from build123d import *

# Parameters (mm, degrees)
SKETCH1_R           = 1.135
SKETCH1_R_2         = 1.054
BOSS_EXTRUDE1_DEPTH = 3
SKETCH2_R           = 0.65
CUT_EXTRUDE1_DEPTH  = 23.736281859
SKETCH4_R           = 0.25
CUT_EXTRUDE3_DEPTH  = 0.25


with BuildPart() as part:
    # Sketch1 → Boss-Extrude1 (new body)
    with BuildSketch(Plane(origin=(0, 0, 0), x_dir=(1, 0, 0), z_dir=(0, 1, 0))):
        with BuildLine():
            Line((0, 0), (9.035898385, 0))
            ThreePointArc((9.035898385, 0), (10.767949192, 1), (10.767949192, 3))
            Line((10.767949192, 3), (1.732050808, 18.650635095))
            ThreePointArc((1.732050808, 18.650635095), (0, 19.650635095), (-1.732050808, 18.650635095))
            Line((-1.732050808, 18.650635095), (-10.767949192, 3))
            ThreePointArc((-10.767949192, 3), (-10.767949192, 1), (-9.035898385, 0))
            Line((-9.035898385, 0), (0, 0))
        make_face()
        with Locations(Location((0, 17.650635095, 0), (0, 0, 270))):
            Circle(SKETCH1_R, mode=Mode.SUBTRACT)
        with Locations(Location((-9.035898385, 2, 0), (0, 0, 270))):
            Circle(SKETCH1_R, mode=Mode.SUBTRACT)
        with Locations(Location((9.035898385, 2, 0), (0, 0, 270))):
            Circle(SKETCH1_R_2, mode=Mode.SUBTRACT)
    extrude(amount=BOSS_EXTRUDE1_DEPTH)

    # Sketch2 → Cut-Extrude1 (cut, through all)
    with BuildSketch(Plane(origin=(0, 3, 0), x_dir=(1, 0, 0), z_dir=(0, 1, 0))):
        with Locations(Location((0, 2.5, 0), (0, 0, 270))):
            Circle(SKETCH2_R)
    extrude(amount=-CUT_EXTRUDE1_DEPTH, mode=Mode.SUBTRACT)

    # Sketch4 → Cut-Extrude3 (cut)
    with BuildSketch(Plane(origin=(0, 3, 0), x_dir=(1, 0, 0), z_dir=(0, 1, 0))):
        with Locations(Location((0, 9.930442918, 0), (0, 0, 270))):
            Circle(SKETCH4_R)
    extrude(amount=-CUT_EXTRUDE3_DEPTH, mode=Mode.SUBTRACT)


solid = part.part
Here's how the part is built. I have some questions about the finished solid (model axes, mm). Coordinates: 2 decimals unless noted, no trailing zeros. Order: outer loops, then holes, each group sorted by start corner. A loop starts at its lowest first (then second) coordinate and runs counter-clockwise, first axis right, second up. Notation, with made-up numbers: M 13,11.25 L 21,11.25 A17 cw 21,16.25 Z; hole C 85.5,-4 d5. An arc over 180 degrees is marked long. Answer as CSV lines item,"result". Start each with the question number.
1. I need wall thicknesses on line 1 (X direction, y = 0.75, z = -2); line 2 (X direction, y = 1.35, z = -2.25); line 3 (X direction, y = 2.85, z = -18). Which ranges of each line are inside material? Lowest first, please. Write a range as [from, to].
2. We'd pull the mould along X, two halves only. Please class faces 1 (the flat face through (0, 1, 0)), 2 (the cylindrical face through (0.2, 1.52, -1.88)), 3 (the cylindrical face through (0.03, 1.48, -19.65)): released by +X, released by -X, zero draft, split by the parting line, or undercut.
3. For pin 1 (1.4 mm diameter, centred on x = 0, z = -17.65, fed in from -Y), with a flat end and sliding along its axis, tell me the tip position at first contact or that it passes through.
4. I want a section at C-C, the plane z = -17.5. Write out the boundary of the cut face in (x, y).
5. I want a section at A-A, the plane x = 0. Write out the boundary of the cut face in (y, z), and give its area (3 significant figures).
6. I want a section at B-B, the plane y = 0.45. Write out the boundary of the cut face in (x, z) (3 decimals).
7. I want a section at D-D, the plane x = 9.5. Write out the boundary of the cut face in (y, z).
Recorded:
1,line 1,"x = [-11.04, -10.17], [-7.9, -0.42], [0.42, 7.98], [10.09, 11.04]"
1,line 2,"x = [-11.02, -10.14], [-7.93, -0.6], [0.6, 8.01], [10.06, 11.02]"
1,line 3,"x = [-2.11, -1.08], [1.08, 2.11]"
2,face 1,"zero draft"
2,face 2,"undercut"
2,face 3,"split by the parting line"
3,pin 1,"passes through"
4,outline,"M -2.4,0 L -1.12,0 L -1.12,3 L -2.4,3 Z; M 1.12,0 L 2.4,0 L 2.4,3 L 1.12,3 Z"
5,outline,"M 0,-19.65 L 3,-19.65 L 3,-18.79 L 0,-18.79 Z; M 0,-16.52 L 3,-16.52 L 3,-10.18 L 2.75,-10.18 L 2.75,-9.68 L 3,-9.68 L 3,-3.15 L 0,-3.15 Z; M 0,-1.85 L 3,-1.85 L 3,0 L 0,0 Z"
5,area,"48.1 mm2"
6,outline,"M -10.768,-3 L -1.732,-18.651 A2 ccw 1.732,-18.651 L 10.768,-3 A2 ccw 9.036,0 L -9.036,0 A2 ccw Z; hole C -9.036,-2 d2.27; hole C 0,-17.651 d2.27; hole C 0,-2.5 d1.3; hole C 9.036,-2 d2.108"
7,outline,"M 0,-5.2 L 3,-5.2 L 3,-2.95 L 0,-2.95 Z; M 0,-1.05 L 3,-1.05 L 3,-0.05 L 0,-0.05 Z"
